Check sheet for the modelled part. Datum: model origin and axes. Units: mm. Face numbers are marked on the shaded views. A direction names the side the tool comes from. Round coordinates to 2 decimals unless told otherwise and drop trailing zeros. Loops run counter-clockwise (first coordinate to the right, second up) from the corner with the lowest first, then second, coordinate; pieces in that order, holes last. Notation, with made-up numbers: M 22,85 L 73,85 A27 cw 73,102 Z; hole C 53,24 d10. An arc over 180 degrees is marked long. One line per question, with ' | ' between items. Start each with the question number.
(1) Section check B-B (y = -13). Record the boundary of the cut face in (x, z), and give its area (3 significant figures).
(2) Tool access check on the marked faces 1, 2, 3 and 4. Record the directions out of +Z, -Z, +X, -X, +Y, -Y that give a thin tool (end or side, any length) a straight path to the whole face; none if there is none.
(3) Section check C-C (x = -0.5). Record the boundary of the cut face in (y, z).
(4) Thickness scan on probe 1 along Y at (x, z) = (7.5, 1.4); probe 2 along X at (y, z) = (19.5, 4.3); probe 3 along Y at (x, z) = (1.5, 0.55). Record the ranges inside material, lowest first. Write a range as [from, to].
(5) Section check A-A (z = 2.7). Record the boundary of the cut face in (x, y).
(6) Draft check along Y on the marked faces 5, 6 and 7. Enter one of: +Y half, -Y half, draft (parallel to the pull), parting line (faces both ways), or undercut.
(7) Section check D-D (y = -28). Record the boundary of the cut face in (x, z).
(8) Go/stop test with flat-tipped pins: P1, Ø3, axis at x = -10.5, z = 2.5, coming from the -Y side; P2, Ø3, axis at x = -8, y = 12.5, coming from the +Z side; P3, Ø6.5, axis at x = 7.5, y = -28, coming from the -Z side; P4, Ø1.4, axis at y = -13, z = 3.5, coming from the +X side. Record where each tip stops, or that it passes through.
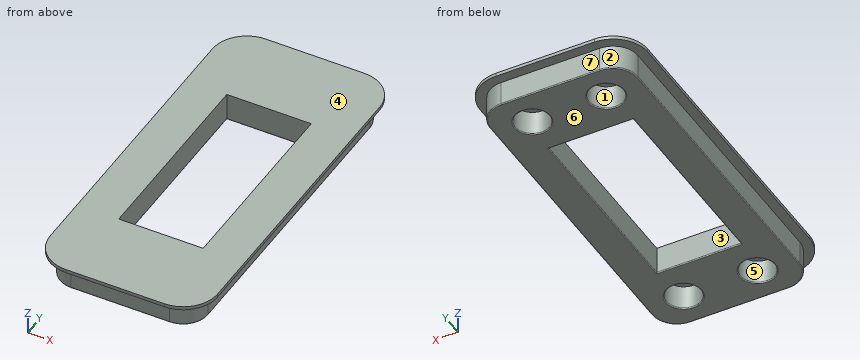
```python
from build123d import *

# Parameters (mm, degrees)
SKETCH4_W           = 30
SKETCH4_H           = 70
SKETCH4_R           = 3.5
SKETCH4_W_2         = 17.142857142
SKETCH4_H_2         = 40
BOSS_EXTRUDE1_DEPTH = 5
SKETCH5_W           = 34
SKETCH5_H           = 74
SKETCH5_W_2         = 30
SKETCH5_H_2         = 70
SKETCH5_R           = 3.5
SKETCH5_W_3         = 17.142857142
SKETCH5_H_3         = 40
BOSS_EXTRUDE2_DEPTH = 0.7
FILLET1_R           = 5
FILLET2_R           = 0.2
FILLET3_R           = 7


with BuildPart() as part:
    # Sketch4 → Boss-Extrude1 (new body)
    with BuildSketch(Plane.XY):
        Rectangle(SKETCH4_W, SKETCH4_H)
        with Locations((7.5, 28)):
            Circle(SKETCH4_R, mode=Mode.SUBTRACT)
        with Locations((-7.5, 28)):
            Circle(SKETCH4_R, mode=Mode.SUBTRACT)
        with Locations((7.5, -28)):
            Circle(SKETCH4_R, mode=Mode.SUBTRACT)
        with Locations((-7.5, -28)):
            Circle(SKETCH4_R, mode=Mode.SUBTRACT)
        Rectangle(SKETCH4_W_2, SKETCH4_H_2, mode=Mode.SUBTRACT)
    extrude(amount=BOSS_EXTRUDE1_DEPTH)

    # Sketch5 → Boss-Extrude2 (add)
    # profile 1 of 6: a face of its own
    with BuildSketch(Plane.XY.offset(5)):
        Rectangle(SKETCH5_W, SKETCH5_H)
        Rectangle(SKETCH5_W_2, SKETCH5_H_2, mode=Mode.SUBTRACT)
    # profile 2 of 6: a face of its own
    with BuildSketch(Plane.XY.offset(5)):
        Rectangle(SKETCH5_W_2, SKETCH5_H_2)
        with Locations((-7.5, 28)):
            Circle(SKETCH5_R, mode=Mode.SUBTRACT)
        with Locations((-7.5, -28)):
            Circle(SKETCH5_R, mode=Mode.SUBTRACT)
        with Locations((7.5, -28)):
            Circle(SKETCH5_R, mode=Mode.SUBTRACT)
        with Locations((7.5, 28)):
            Circle(SKETCH5_R, mode=Mode.SUBTRACT)
        Rectangle(SKETCH5_W_3, SKETCH5_H_3, mode=Mode.SUBTRACT)
    # profile 3 of 6: a face of its own
    with BuildSketch(Plane.XY.offset(5)):
        with Locations((7.5, -28)):
            Circle(SKETCH5_R)
    # profile 4 of 6: a face of its own
    with BuildSketch(Plane.XY.offset(5)):
        with Locations((-7.5, -28)):
            Circle(SKETCH5_R)
    # profile 5 of 6: a face of its own
    with BuildSketch(Plane.XY.offset(5)):
        with Locations((7.5, 28)):
            Circle(SKETCH5_R)
    # profile 6 of 6: a face of its own
    with BuildSketch(Plane.XY.offset(5)):
        with Locations((-7.5, 28)):
            Circle(SKETCH5_R)
    extrude(amount=BOSS_EXTRUDE2_DEPTH)

    # Fillet1
    fillet1_edges = [part.edges().sort_by_distance(p)[0] for p in [
        (-15, 35, 2.5),
        (15, 35, 2.5),
        (15, -35, 2.5),
        (-15, -35, 2.5),
    ]]
    fillet(fillet1_edges, radius=FILLET1_R)

    # Fillet2
    fillet2_edges = [part.edges().sort_by_distance(p)[0] for p in [
        (-11, -28, 0),
        (4, -28, 0),
        (8.571428571, 0, 0),
        (0, 20, 0),
        (-8.571428571, 0, 0),
        (0, -20, 0),
        (-11, 28, 0),
        (4, 28, 0),
        (15, 0, 0),
        (-15, 0, 0),
        (0, 35, 0),
        (0, -35, 0),
        (13.535533906, 33.535533906, 0),
        (-13.535533906, 33.535533906, 0),
        (-13.535533906, -33.535533906, 0),
        (13.535533906, -33.535533906, 0),
    ]]
    fillet(fillet2_edges, radius=FILLET2_R)

    # Fillet3
    fillet3_edges = [part.edges().sort_by_distance(p)[0] for p in [
        (17, 37, 5.35),
        (-17, 37, 5.35),
        (-17, -37, 5.35),
        (17, -37, 5.35),
    ]]
    fillet(fillet3_edges, radius=FILLET3_R)


solid = part.part
```
The answers:
1) outline: M -17,5 L -15,5 L -15,0.2 A0.2 ccw -14.8,0 L -8.77,0 A0.2 ccw -8.57,0.2 L -8.57,5.7 L -17,5.7 Z; M 8.57,0.2 A0.2 ccw 8.77,0 L 14.8,0 A0.2 ccw 15,0.2 L 15,5 L 17,5 L 17,5.7 L 8.57,5.7 Z | area: 76.1 mm²
2) face 1: -Z | face 2: -Z, -X, +Y | face 3: +Z, -Z | face 4: +Z, +X, -X, +Y, -Y
3) outline: M -37,5 L -35,5 L -35,0.2 A0.2 ccw -34.8,0 L -20.2,0 A0.2 ccw -20,0.2 L -20,5.7 L -37,5.7 Z; M 20,0.2 A0.2 ccw 20.2,0 L 34.8,0 A0.2 ccw 35,0.2 L 35,5 L 37,5 L 37,5.7 L 20,5.7 Z
4) probe 1: [-35, -31.5], [-24.5, -20], [20, 24.5], [31.5, 35] | probe 2: [-15, -8.57], [8.57, 15] | probe 3: [-35, -20], [20, 35]
5) outline: M -15,-30 A5 ccw -10,-35 L 10,-35 A5 ccw 15,-30 L 15,30 A5 ccw 10,35 L -10,35 A5 ccw -15,30 Z; hole C -7.5,-28 d7; hole C -7.5,28 d7; hole M -8.57,-20 L 8.57,-20 L 8.57,20 L -8.57,20 Z; hole C 7.5,-28 d7; hole C 7.5,28 d7
6) face 5: undercut | face 6: draft | face 7: +Y half
7) outline: M -17,5 L -15,5 L -15,0.2 A0.2 ccw -14.8,0 L -11.2,0 A0.2 ccw -11,0.2 L -11,5 L -4,5 L -4,0.2 A0.2 ccw -3.8,0 L 3.8,0 A0.2 ccw 4,0.2 L 4,5 L 11,5 L 11,0.2 A0.2 ccw 11.2,0 L 14.8,0 A0.2 ccw 15,0.2 L 15,5 L 17,5 L 17,5.7 L -17,5.7 Z
8) P1: y = -35 | P2: z = 5.7 | P3: z = 5 | P4: x = 15
